Design review of the part built by this model. Coordinates are the model's own, in mm. A direction names the side the tool comes from. Coordinates: 2 decimals unless noted, no trailing zeros. Loops run counter-clockwise (first coordinate to the right, second up) from the corner with the lowest first, then second, coordinate; pieces in that order, holes last.
Q1. Draft analysis for pull direction X (two halves, no side actions). For faces 5 (the face through (-84.302, 2, -56)), 6 (the face through (-42, 0, -53)), 7 (the face through (0, 2, -54)), 8 (the face through (-87, 4, -56)), state which applies: released by +X, released by -X, zero draft, split by the parting line, or undercut.
Q2. For P1, Ø1.2, axis at y = 2, z = -45, coming from the +X side; P2, Ø3, axis at x = -45.5, z = -31.5, coming from the -Y side; P3, Ø1.5, axis at x = -77, y = 0.5, coming from the -Z side, all flat-tipped, find the tip position at first contact; note any pin that passes through.
Q3. Add section B-B on z = -11. Give the boundary of the cut face in (x, y).
Q4. Add section C-C on x = -58. Give the boundary of the cut face in (y, z), and give its area (3 significant figures).
Q5. Add section A-A on y = -3.5. Give the boundary of the cut face in (x, z), and give its area (3 significant figures).
Q6. Wall thickness on probe 1 along Y at (x, z) = (-7.5, -19); probe 2 along Z at (x, y) = (-52, -1.5); probe 3 along X at (y, z) = (-4, -97.5): over which ranges is each line inside the solid? List them lowest first.
Q7. Machinability: for faces 1 (the face through (-39.6, -2.46, 6.11)), 2 (the face through (-41.56, 1.97, 10.6)), 3 (the face through (-39.616, 4.986, 13.314)), 4 (the face through (-41.56, 1.97, -119.6)), which of the approach directions +Z, -Z, +X, -X, +Y, -Y give a long, thin tool a straight path to every point of the face, cutting with its end or side? Answer none if there is none.
Autodesk Inventor part; units mm, degrees
ref_plane "YZ Plane" through (0, 0, 0) normal (1, 0, 0) x (0, 1, 0)
ref_plane "XZ Plane" through (0, 0, 0) normal (0, 1, 0) x (-1, 0, 0)
ref_plane "XY Plane" through (0, 0, 0) normal (0, 0, 1) x (1, 0, 0)
sketch "Sketch1" plane through (0, 0, 0) normal (0, 1, 0) x (-1, 0, 0)
  line L0 (0, 0) -> (0, -109)
  line L1 (0, -109) -> (84.3015, -130.5)
  line L2 (84.3015, -130.5) -> (84.3015, 21.5)
  line L3 (0, 0) -> (84.3015, 21.5)
  dimension "d0" = 109
  dimension "d3" = 87
  dimension "d4" = 152
  dimension "d5" = 87
extrude "Extrusion1" add sketch "Sketch1" along normal blind 4
sketch "Sketch2" plane through (0, 0, 0) normal (0, -1, 0) x (1, 0, 0)
  line L0 (0, 0) -> (0, -109)
  line L1 (0, -109) -> (-5, -109)
  line L2 (-4.8329, -103.795) -> (-4.8329, -3.205)
  line L3 (-5, 0) -> (0, 0)
  line L4 (0, 0) -> (0, -109)
  line L5 (0, -109) -> (-84.3015, -130.5)
  line L6 (-84.3015, -130.5) -> (-74.4446, -130.5)
  line L7 (-79.3015, 21.5) -> (-84.3015, 21.5)
  line L8 (-84.3015, 21.5) -> (-84.3015, -130.5)
  line L9 (-84.3015, -130.5) -> (0, -109)
  line L10 (0, -109) -> (-1.2356, -104.1551)
  line L11 (-85.5402, -125.6434) -> (-84.3015, -130.5)
  line L12 (-84.3015, -130.5) -> (-84.3015, 21.5)
  line L13 (0, 0) -> (-84.3015, 21.5)
  line L14 (-84.3015, 21.5) -> (-85.5372, 16.6551)
  line L15 (-1.4353, -5.628) -> (0, 0)
  line L16 (-74.4446, -130.5) -> (-74.4446, -127.9861)
  line L17 (-4.8329, -103.795) -> (-74.2654, -121.5028)
  line L18 (-84.3015, -125.3275) -> (-85.5402, -125.6434)
  line L19 (-85.5372, 16.6551) -> (-84.3015, 16.34)
  line L20 (-74.2654, 14.5028) -> (-4.8329, -3.205)
  line L21 (-79.3015, 20.2248) -> (-79.3015, 21.5)
  line L22 (-79.3015, 15.8371) -> (-79.3015, -122.7872)
  line L23 (-74.2654, -121.5028) -> (-79.3015, -122.7872)
  line L24 (-74.2654, 14.5028) -> (-79.3015, 15.8371)
  dimension "d9" = 5
  dimension "d10" = 5
  dimension "d11" = 5
  dimension "d12" = 5
extrude "Extrusion2" add sketch "Sketch2" along normal blind 5 draft -10 contours L0 L5 L8 L13
sketch "Sketch3" plane through (0, 4, 0) normal (0, 1, 0) x (1, 0, 0)
  line L0 (0, 34.4959) -> (3, 34.4959) construction
  line L1 (3.8363, -2.2322) -> (3.8363, 112.6381)
  line L2 (-79.382, 43.4403) -> (-76.382, 43.4403) construction
  line L3 (-84.3015, 130.5) -> (-84.3015, -21.5)
  line L4 (-84.3015, 135.1165) -> (3.8363, 112.6381)
  line L5 (0, 109) -> (-84.3015, 130.5)
  line L6 (3.8363, -2.2322) -> (-84.3015, -24.7106)
  line L7 (-84.3015, -21.5) -> (0, 0)
  line L8 (-84.3015, 130.5) -> (-84.3015, 135.1165)
  line L9 (-84.3015, -21.5) -> (-84.3015, -24.7106)
  line L10 (-84.3015, 135.1165) -> (-88.3015, 135.1165)
  line L11 (-88.3015, 135.1165) -> (-88.3015, -24.7106)
  line L12 (-88.3015, -24.7106) -> (-84.3015, -24.7106)
  line L13 (-84.3015, -24.7106) -> (-84.3015, 135.1165)
  dimension "d24" = 4
extrude "Extrusion3" add sketch "Sketch3" along normal blind 2
properties part number "FoodHopperLid"
Entries:
1. face 5: released by -X
1. face 6: undercut
1. face 7: released by +X
1. face 8: zero draft
2. P1: stops at x = 0
2. P2: stops at y = 0
2. P3: stops at z = -128.83
3. outline: (-88.3, 4) - (-84.3, 4) - (-84.3, 0) - (-83.42, -5) - (-80.18, -5) - (-79.3, 0) - (-4.83, 0) - (-3.95, -5) - (-0.88, -5) - (0, 0) - (0, 4) - (3.84, 4) - (3.84, 6) - (-88.3, 6) - close
4. outline: (-5, -122.88) - (0, -123.79) - (4, -123.79) - (4, -128.41) - (6, -128.41) - (6, 18) - (4, 18) - (4, 14.79) - (0, 14.79) - (-5, 13.88) - (-5, 11.26) - (0, 10.35) - (0, -117.35) - (-5, -118.26) - close
4. area: 892 mm2
5. outline: (-83.68, -129.71) - (-0.62, -108.52) - (-0.62, -0.48) - (-83.68, 20.71) - close; hole (-79.92, -123.58) - (-74.11, -122.1) - (-4.22, -104.27) - (-4.22, -2.73) - (-74.11, 15.1) - (-79.92, 16.64) - close
5. area: 1,590 mm2
6. probe 1: y = 0 to 6
6. probe 2: z = -121.99 to -116.1, 9.1 to 12.99
6. probe 3: x = -83.6 to -80.01, -4.13 to -0.71
7. face 1: -Y
7. face 2: +Z, +X, -Y
7. face 3: +Z, +X, +Y, -Y
7. face 4: -Z, +X, -Y
